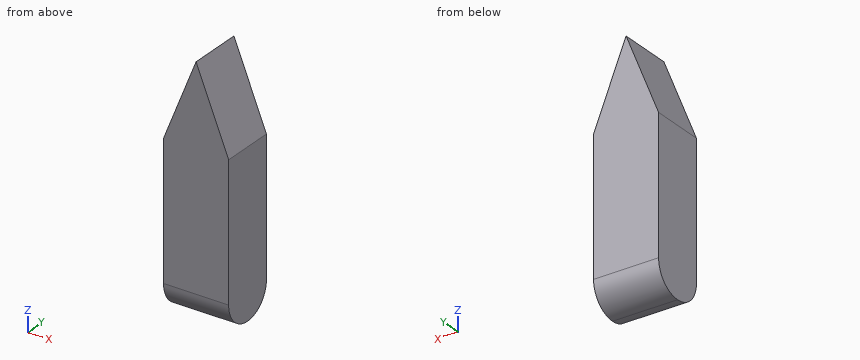
```python
from build123d import *

# Parameters (mm, degrees)
SKETCH_2_W          = 12
SKETCH_2_H          = 10
EXTRUDE_1_DEPTH     = 45
CUT_EXTRUDE_1_DEPTH = 65
CUT_EXTRUDE_2_DEPTH = 65


with BuildPart() as part:
    # 草图2 → 凸台-拉伸1 (new body)
    with BuildSketch(Plane.XY):
        with Locations((6, 5)):
            Rectangle(SKETCH_2_W, SKETCH_2_H)
    extrude(amount=EXTRUDE_1_DEPTH)

    # 草图3 → 切除-拉伸1 (cut)
    with BuildSketch(Plane(origin=(12, 0, 0), x_dir=(0, 0, -1), z_dir=(1, 0, 0))):
        with BuildLine():
            Line((0, 0), (0, 5))
            ThreePointArc((0, 5), (-1.464466094, 1.464466094), (-5, 0))
            Line((-5, 0), (0, 0))
        make_face()
        with BuildLine():
            Line((0, 10), (-5, 10))
            ThreePointArc((-5, 10), (-1.464466094, 8.535533906), (0, 5))
            Line((0, 5), (0, 10))
        make_face()
    extrude(amount=-CUT_EXTRUDE_1_DEPTH, mode=Mode.SUBTRACT)

    # 草图4 → 切除-拉伸2 (cut)
    with BuildSketch(Plane.XZ):
        Polygon((0, 45), (0, 30), (6, 45), align=None)
        Polygon((12, 45), (6, 45), (12, 30), align=None)
    extrude(amount=-CUT_EXTRUDE_2_DEPTH, mode=Mode.SUBTRACT)


solid = part.part
```
Read the model definition and answer for the solid it produces. Units are mm, in the model's axes. Give positions to 0.01 mm unless a question says otherwise; leave off trailing zeros. Order: outer loops, then holes, each group sorted by start corner. A loop starts at its lowest first (then second) coordinate and runs counter-clockwise, first axis right, second up. Notation, with made-up numbers: (56.5, 69.5) -> (93.5, 69.5) arc R29 ccw to (93.5, 107.5) -> close; hole circle Ø4 at (-23, 87). An arc over 180 degrees is marked (long way). One line per item, written item: value. Start each with the question number.
(1) Straight lines are drawn through the part: L1, parallel to X at y = 5, z = 32.5; L2, parallel to X at y = 2, z = 32; L3, parallel to Z at x = 11.5, y = 1.75. For each, find the intervals that lie inside material, in ascending order.
(2) Flat-ended cylindrical pins translate along their axes: P1, Ø4, axis at y = 4.5, z = 27, coming from the -X side; P2, Ø3, axis at y = 2, z = 39, coming from the -X side; P3, Ø1.5, axis at x = 10.5, y = 2.5, coming from the -Z side. Find the tip coordinate at first contact, or state that the pin passes through.
(3) The part is cut by section C-C (z = 36). Determine the outline of the cut face in (x, y).
(4) The part is cut by section B-B (y = 3). Determine the outline of the cut face in (x, z), and give its area (3 significant figures).
(5) The part is cut by section A-A (x = 1.5). Determine the outline of the cut face in (y, z).
Taken from the geometry:
1. L1: 1 to 11
1. L2: 0.8 to 11.2
1. L3: 1.2 to 31.25
2. P1: x = 0
2. P2: x = 3
2. P3: z = 0.32
3. outline: (2.4, 0) -> (9.6, 0) -> (9.6, 10) -> (2.4, 10) -> close
4. outline: (0, 0.42) -> (12, 0.42) -> (12, 30) -> (6, 45) -> (0, 30) -> close
4. area: 445 mm^2
5. outline: (0, 5) arc R5 ccw to (10, 5) -> (10, 33.75) -> (0, 33.75) -> close
